Work out the finished part from the listing and answer in its coordinate system (mm). Face numbers are marked on the shaded views. A direction names the side the tool comes from. Coordinates: 2 decimals unless noted, no trailing zeros. Loops run counter-clockwise (first coordinate to the right, second up) from the corner with the lowest first, then second, coordinate; pieces in that order, holes last. Notation, with made-up numbers: M 42,34.25 L 58,34.25 A22 cw 58,48.25 Z; hole C 50.25,-37.75 d6. An arc over 180 degrees is marked long. Write each question's results on one line, items separated by ' | '.
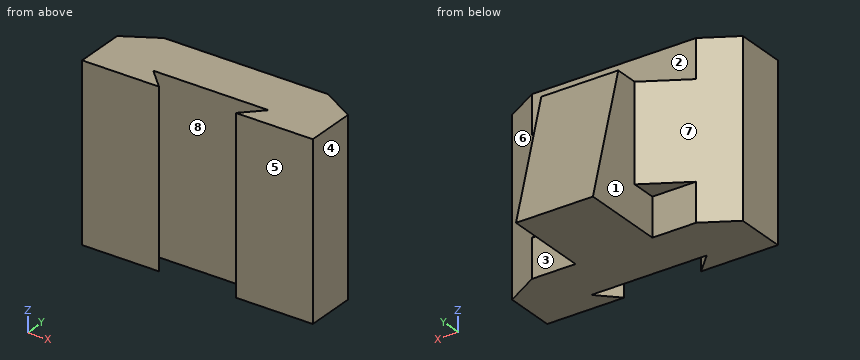
Autodesk Inventor part; units mm, degrees
ref_plane "YZ Plane" through (0, 0, 0) normal (1, 0, 0) x (0, 1, 0)
ref_plane "XZ Plane" through (0, 0, 0) normal (0, 1, 0) x (-1, 0, 0)
ref_plane "XY Plane" through (0, 0, 0) normal (0, 0, 1) x (1, 0, 0)
sketch "Sketch1" plane through (0, 0, 0) normal (0, 0, 1) x (1, 0, 0)
  line L0 (0, 0) -> (20, 0)
  line L1 (20, 0) -> (15, 5)
  line L2 (15, 5) -> (45, 5)
  line L3 (45, 5) -> (40, 0)
  line L4 (40, 0) -> (60, 0)
  line L5 (60, 0) -> (60, 13)
  line L6 (0, 0) -> (0, 13)
  line L7 (20, 24.547) -> (20, 40)
  line L8 (20, 40) -> (40, 40)
  line L9 (40, 40) -> (40, 24.547)
  line L10 (60, 13) -> (40, 24.547)
  line L11 (20, 24.547) -> (0, 13)
extrude "Extrusion1" add sketch "Sketch1" along normal blind 45
sketch "Sketch2" plane through (0, 0, 45) normal (0, 0, 1) x (1, 0, 0)
  line L0 (20, 24.547) -> (0, 13)
  line L1 (8.6603, 18) -> (51.3397, 18)
  line L2 (60, 13) -> (40, 24.547)
  line L3 (8.6603, 18) -> (20, 24.547)
  line L4 (20, 40) -> (20, 24.547)
  line L5 (20, 24.547) -> (20, 40)
  line L6 (20, 40) -> (40, 40)
  line L7 (40, 40) -> (40, 24.547)
  line L8 (40, 24.547) -> (40, 40)
  line L9 (40, 24.547) -> (51.3397, 18)
  point P0 (0, 0)
extrude "Extrusion2" cut sketch "Sketch2" against normal blind 10
sketch "Sketch3" plane through (40, 24.547, 0) normal (1, 0, 0) x (0, 0, -1)
  line L0 (0, 0) -> (0, 15.453)
  line L1 (0, 15.453) -> (37.2699, 15.453) construction
  line L2 (-35, 0) -> (-35, 15.453)
  line L3 (-35, 15.453) -> (0, 15.453)
  line L4 (0, 15.453) -> (-35, 6.0748)
  line L5 (-35, 6.0748) -> (-35, 15.453)
  point P0 (0, -24.547)
extrude "Extrusion3" cut sketch "Sketch3" against normal blind 20
sketch "Sketch4" plane through (60, 0, 0) normal (1, 0, 0) x (0, 0, -1)
  line L0 (0, 18) -> (-10, 18)
  line L1 (-10, 18) -> (-10, 24.547)
  line L2 (0, 24.547) -> (-35, 24.547)
  line L3 (0, 24.547) -> (0, 40)
  line L4 (-10, 24.547) -> (0, 24.547)
  line L5 (0, 24.547) -> (0, 18)
  point P0 (0, 0)
extrude "Extrusion4" cut sketch "Sketch4" against normal blind 20
sketch "Sketch5" plane through (0, 0, 0) normal (-1, 0, 0) x (0, 0, 1)
  line L0 (10, 18) -> (10, 24.547)
  line L1 (10, 18) -> (10, 24.547)
  line L2 (0, 24.547) -> (35, 24.547)
  line L3 (10, 24.547) -> (0, 24.547)
  line L4 (0, 24.547) -> (0, 18)
  line L5 (0, 24.547) -> (0, 13)
  line L6 (0, 18) -> (10, 18)
  line L7 (10, 18) -> (0, 18)
  point P0 (0, 0)
extrude "Extrusion5" cut sketch "Sketch5" against normal blind 20
properties part number "P3-15"
1) Find section C-C, the plane z = 34. Give the vertices of the cut face in (x, y), and give its area (3 significant figures).
Check result:
outline: M 0,0 L 20,0 L 15,5 L 45,5 L 40,0 L 60,0 L 60,13 L 40,24.55 L 40,30.89 L 20,30.89 L 20,24.55 L 0,13 Z | area: 1,240 mm^2
2) Find section D-D, the plane y = 20. Give the vertices of the cut face in (x, z).
Check result:
outline: M 12.12,10 L 20,10 L 20,0 L 40,0 L 40,10 L 47.88,10 L 47.88,35 L 12.12,35 Z
3) Given pin 1 Ø3 at (y, z) = (20.5, 30.5) entering from +X; pin 2 Ø2 at (x, y) = (17, 20) entering from -Z; pin 3 Ø5 at (x, z) = (16, 6) entering from +Y, each flat-ended and moving along its own axis, determine where each tip first touches the part or whether it passes through.
Check result:
pin 1: x = 49.61 | pin 2: z = 10 | pin 3: y = 18
4) For a pull along X with two mould halves and no side action, classify the marked faces 5, 6, 7 and 8 as released by +X, released by -X, zero draft, split by the parting line, or undercut.
Check result:
face 5: zero draft | face 6: released by +X | face 7: released by -X | face 8: undercut
5) Straight lines are drawn through the part: probe 1 along X at (y, z) = (31, 22); probe 2 along X at (y, z) = (18, 29); probe 3 along Y at (x, z) = (47.5, 6). For each, find the intervals that lie inside material, in ascending order. Write a range as [from, to].
Check result:
probe 1: [20, 40] | probe 2: [8.66, 51.34] | probe 3: [0, 18]
6) Which of the six approach directions +Z, -Z, +X, -X, +Y, -Y give full straight-line access (tool end or side, diameter ignored) to the marked faces 1, 2, 3 and 4?
Check result:
face 1: -Z, -X, +Y | face 2: +Z, +X, -X, +Y | face 3: -Z, +X, +Y | face 4: +Z, -Z, +X, +Y, -Y
7) Find section A-A, the plane y = 3. Give the vertices of the cut face in (x, z).
Check result:
outline: M 0,0 L 17,0 L 17,45 L 0,45 Z; M 43,0 L 60,0 L 60,45 L 43,45 Z
8) Find section B-B, the plane x = 19. Give the vertices of the cut face in (y, z), and give its area (3 significant figures).
Check result:
outline: M 0,0 L 1,0 L 1,45 L 0,45 Z; M 5,0 L 18,0 L 18,10 L 23.97,10 L 23.97,35 L 18,35 L 18,45 L 5,45 Z | area: 779 mm^2
